Part model, mm, in its own coordinate system. A direction names the side the tool comes from. Coordinates: 2 decimals unless noted, no trailing zeros. Write each loop counter-clockwise with the first axis right and the second up, starting at its lowest first coordinate (ties: lowest second). Pieces come first, ordered by that corner, then holes. Notation, with made-up numbers: (3.25, 6) -> (44.25, 6) arc R18 cw to (44.25, 38) -> close; hole circle Ø8 at (-34, 0.5). An arc over 180 degrees is marked (long way). Write item = value, one per line.
from build123d import *

# Parameters (mm, degrees)
F0_R     = 14.5
F0_R_2   = 11.5
F0_R_3   = 9.15
F0_R_4   = 4.25
F1_DEPTH = 10
F2_DEPTH = 1.5
F3_SIZE  = 0.5


with BuildPart() as f1:
    # F0 (on Top) → F1 (new body)
    with BuildSketch(Plane.XY):
        Circle(F0_R)
        Circle(F0_R_2, mode=Mode.SUBTRACT)
        Circle(F0_R_2)
        Circle(F0_R_3, mode=Mode.SUBTRACT)
        Circle(F0_R_3)
        Circle(F0_R_4, mode=Mode.SUBTRACT)
    extrude(amount=-F1_DEPTH)

    # F0 (on Top) → F2 (join)
    with BuildSketch(Plane.XY):
        Circle(F0_R_2)
        Circle(F0_R_3, mode=Mode.SUBTRACT)
    extrude(amount=F2_DEPTH)

    # F3
    f3_edges = [f1.edges().sort_by_distance(p)[0] for p in [
        (-11.5, 0, 1.5),
        (-9.15, 0, 1.5),
    ]]
    chamfer(f3_edges, length=F3_SIZE)


solid = f1.part
Q1. Saw through at C-C on z = -2.5. Give the cut face in (x, y).
Model answer:
outline = circle Ø29 at (0, 0); hole circle Ø8.5 at (0, 0)
Q2. Saw through at A-A on x = 0. Give the cut face in (y, z).
Model answer:
outline = (-14.5, -10) -> (-4.25, -10) -> (-4.25, 0) -> (-9.15, 0) -> (-9.15, 1) -> (-9.65, 1.5) -> (-11, 1.5) -> (-11.5, 1) -> (-11.5, 0) -> (-14.5, 0) -> close; (4.25, -10) -> (14.5, -10) -> (14.5, 0) -> (11.5, 0) -> (11.5, 1) -> (11, 1.5) -> (9.65, 1.5) -> (9.15, 1) -> (9.15, 0) -> (4.25, 0) -> close
Q3. Which spindle directions (+Z, -Z, +X, -X, +Y, -Y) get a long thin tool onto all of the face, cutting with end or side? Do faces 1 (the face through (2.285, 3.584, -4.93)), 2 (the face through (-1.5, 11.4, 0.5)). Say none if no direction does.
Model answer:
face_1 = +Z, -Z
face_2 = +Z
Q4. Probe line 1 (Y direction, x = 0, z = -6.5); line 2 (Y direction, x = 0, z = 0.6); line 3 (Z direction, x = -5, y = 4.5). List the from-to ranges inside material, lowest first. Write a range as from..to.
Model answer:
line_1 = -14.5..-4.25, 4.25..14.5
line_2 = -11.5..-9.15, 9.15..11.5
line_3 = -10..0
Q5. Mould opens along Y. For faces 3 (the face through (3, 3.4, -10)), 4 (the face through (2, -4, 0)), 5 (the face through (6.691, -12.864, -4.93)) say: released by +Y, released by -Y, zero draft, split by the parting line, or undercut.
Model answer:
face_3 = zero draft
face_4 = undercut
face_5 = split by the parting line
Q6. Pin check, flat tips, straight feed: pin 1 (4 mm diameter, centred on x = 2.5, y = 2, fed in from +Z); pin 2 (1 mm diameter, centred on x = 11, y = 10.5, fed in from -Z); pin 3 (6 mm diameter, centred on y = 9.5, z = -3.5, fed in from -X); pin 4 (5 mm diameter, centred on y = 3, z = -7, fed in from -X). Stop position of each tip, or through.
Model answer:
pin_1 = 0
pin_2 = through
pin_3 = -12.96
pin_4 = -14.49
